Work out the finished part from the listing and answer in its coordinate system (mm). A direction names the side the tool comes from. Round coordinates to 2 decimals unless told otherwise and drop trailing zeros. Write each loop counter-clockwise with the first axis right and the second up, starting at its lowest first coordinate (ties: lowest second). Pieces come first, ordered by that corner, then holes.
1. Flat-ended cylindrical pins translate along their axes: pin 1 Ø10 at (y, z) = (67.5, 14.5) entering from +X; pin 2 Ø3 at (x, y) = (11, 97) entering from +Z; pin 3 Ø15.5 at (x, z) = (0.5, 2.5) entering from -Y; pin 4 Ø5 at (x, y) = (-11, 12.5) entering from -Z. Find the tip coordinate at first contact, or state that the pin passes through.
2. A tool of negligible diameter and unlimited length cuts with its end or side. For faces 1 (the face through (-20.93, 71.86, 17.35)), 2 (the face through (14.39, 89, -8)), 3 (the face through (5.437, 0.493, -17.264)), from which of +Z, -Z, +X, -X, +Y, -Y can it reach the whole face along a straight path? Write none if from no direction.
3. Straight lines are drawn through the part: probe 1 along X at (y, z) = (92.15, -16); probe 2 along Y at (x, z) = (-9.5, -19); probe 3 along X at (y, z) = (-3, 0). For each, find the intervals that lie inside material, in ascending order.
4. Find section D-D (y = 98). Write down the section's boundary in (x, z), and give its area (3 significant figures).
5. Find section C-C (z = 0). Count the separate pieces of the cut face and the enclosed holes in it, and give its area (3 significant figures).
6. Find section A-A (y = 79.5). Write down the section's boundary in (x, z), and give its area (3 significant figures).
7. Determine the mould class of faces 4 (the face through (2, 91, -9)), 5 (the face through (22, 83, -6)), 6 (the face through (-5, 77.5, -16)) for opening direction X: pulls with the +X half, pulls with the -X half, needs draft (parallel to the pull), parting line crosses it, or undercut.
8. Find section B-B (y = 13.5). Write down the section's boundary in (x, z).
```python
from build123d import *

# Parameters (mm, degrees)
SKETCH_1_R           = 18.6
EXTRUDE_1_DEPTH      = 15
SKETCH_2_R           = 19.1
EXTRUDE_2_DEPTH      = 43
FILLET_4_R           = 1
SKETCH_3_R           = 18.1
CUT_EXTRUDE_1_DEPTH  = 1
SKETCH_4_R           = 7.3
EXTRUDE_3_DEPTH      = 5.7
FILLET_5_R           = 1
SKETCH_5_R           = 4
CUT_EXTRUDE_2_DEPTH  = 2
SKETCH_6_R           = 2.25
EXTRUDE_4_DEPTH      = 2
SKETCH_7_R           = 7
EXTRUDE_5_DEPTH      = 4.1
SKETCH_8_R           = 6.5
CUT_EXTRUDE_3_DEPTH  = 2.6
SKETCH_9_R           = 2.5
EXTRUDE_6_DEPTH      = 3
SKETCH_10_R          = 5
EXTRUDE_7_DEPTH      = 19
SKETCH_12_W          = 44
SKETCH_12_H          = 57
EXTRUDE_8_DEPTH      = 4
SKETCH_13_R          = 3
EXTRUDE_9_DEPTH      = 20
SKETCH_14_R          = 3
EXTRUDE_10_DEPTH     = 20
SKETCH_15_R          = 3
EXTRUDE_11_DEPTH     = 20
SKETCH_16_R          = 3
EXTRUDE_12_DEPTH     = 20
SKETCH_17_W          = 44
SKETCH_17_H          = 57
EXTRUDE_13_DEPTH     = 3
SKETCH_21_R          = 6.5
SKETCH_21_R_2        = 2.5
CUT_EXTRUDE_5_DEPTH  = 4
CUT_EXTRUDE_START    = -4
SKETCH_22_R          = 7
CUT_EXTRUDE_6_DEPTH  = 4
SKETCH_23_R          = 5.5
SKETCH_23_R_2        = 4.5
EXTRUDE_14_DEPTH     = 0.1
SKETCH_24_R          = 4
EXTRUDE_15_DEPTH     = 10
SKETCH_25_R          = 5
EXTRUDE_16_DEPTH     = 3.5
SKETCH_28_R          = 10.9
EXTRUDE_22_DEPTH     = 2
SKETCH_29_R          = 4
EXTRUDE_23_DEPTH     = 4.5
EXTRUDE_START        = 0.1
SKETCH_31_R          = 5.5
SKETCH_31_R_2        = 4.5
EXTRUDE_25_DEPTH     = 0.1
EXTRUDE_26_DEPTH     = 9
CUT_EXTRUDE_7_DEPTH  = 9
CUT_EXTRUDE_8_DEPTH  = 9
SKETCH_39_R          = 2.75
EXTRUDE_27_DEPTH     = 15
CUT_EXTRUDE_9_DEPTH  = 9
SKETCH_41_W          = 1
SKETCH_41_H          = 1
CUT_EXTRUDE_10_DEPTH = 9
SKETCH_42_W          = 1
SKETCH_42_H          = 1
CUT_EXTRUDE_11_DEPTH = 9
FILLET_6_R           = 0.01
FILLET_7_R           = 0.1
SKETCH_43_R          = 7.5
SKETCH_43_R_2        = 7
CUT_EXTRUDE_12_DEPTH = 3
SKETCH_44_R          = 30
EXTRUDE_28_DEPTH     = 5


with BuildPart() as part:
    # ｽｹｯﾁ1 → ﾎﾞｽ - 押し出し1 (new body)
    with BuildSketch(Plane(origin=(0, 0, 0), x_dir=(1, 0, 0), z_dir=(0, 1, 0))):
        with Locations(Location((0, 0, 0), (0, 0, 270))):
            Circle(SKETCH_1_R)
    extrude(amount=EXTRUDE_1_DEPTH)

    # ｽｹｯﾁ2 → ﾎﾞｽ - 押し出し2 (add)
    with BuildSketch(Plane(origin=(0, 15, 0), x_dir=(1, 0, 0), z_dir=(0, 1, 0))):
        with Locations(Location((0, 0, 0), (0, 0, 270))):
            Circle(SKETCH_2_R)
    extrude(amount=EXTRUDE_2_DEPTH)

    # ﾌｨﾚｯﾄ4
    fillet_4_edges = [part.edges().sort_by_distance(p)[0] for p in [
        (0, 58, -19.1),
    ]]
    fillet(fillet_4_edges, radius=FILLET_4_R)

    # ｽｹｯﾁ3 → ｶｯﾄ - 押し出し1 (cut)
    with BuildSketch(Plane.XZ):
        with Locations(Location((0, 0, 0), (0, 0, 270))):
            Circle(SKETCH_3_R)
    extrude(amount=-CUT_EXTRUDE_1_DEPTH, mode=Mode.SUBTRACT)

    # ｽｹｯﾁ4 → ﾎﾞｽ - 押し出し3 (add)
    with BuildSketch(Plane.XZ.offset(-1)):
        with Locations(Location((0, 0, 0), (0, 0, 270))):
            Circle(SKETCH_4_R)
    extrude(amount=EXTRUDE_3_DEPTH)

    # ﾌｨﾚｯﾄ5
    fillet_5_edges = [part.edges().sort_by_distance(p)[0] for p in [
        (0, -4.7, 7.3),
    ]]
    fillet(fillet_5_edges, radius=FILLET_5_R)

    # ｽｹｯﾁ5 → ｶｯﾄ - 押し出し2 (cut)
    with BuildSketch(Plane.XZ.offset(4.7)):
        with Locations(Location((0, 0, 0), (0, 0, 270))):
            Circle(SKETCH_5_R)
    extrude(amount=-CUT_EXTRUDE_2_DEPTH, mode=Mode.SUBTRACT)

    # ｽｹｯﾁ6 → ﾎﾞｽ - 押し出し4 (add)
    with BuildSketch(Plane.XZ.offset(2.7)):
        with Locations(Location((0, 0, 0), (0, 0, 270))):
            Circle(SKETCH_6_R)
    extrude(amount=EXTRUDE_4_DEPTH)

    # ｽｹｯﾁ7 → ﾎﾞｽ - 押し出し5 (add)
    with BuildSketch(Plane(origin=(0, 58, 0), x_dir=(1, 0, 0), z_dir=(0, 1, 0))):
        with Locations(Location((0, 0, 0), (0, 0, 270))):
            Circle(SKETCH_7_R)
    extrude(amount=EXTRUDE_5_DEPTH)

    # ｽｹｯﾁ8 → ｶｯﾄ - 押し出し3 (cut)
    with BuildSketch(Plane(origin=(0, 62.1, 0), x_dir=(1, 0, 0), z_dir=(0, 1, 0))):
        with Locations(Location((0, 0, 0), (0, 0, 270))):
            Circle(SKETCH_8_R)
    extrude(amount=-CUT_EXTRUDE_3_DEPTH, mode=Mode.SUBTRACT)

    # ｽｹｯﾁ9 → ﾎﾞｽ - 押し出し6 (add)
    with BuildSketch(Plane(origin=(0, 59.5, 0), x_dir=(1, 0, 0), z_dir=(0, 1, 0))):
        with Locations(Location((0, 0, 0), (0, 0, 270))):
            Circle(SKETCH_9_R)
    extrude(amount=EXTRUDE_6_DEPTH)

    # ｽｹｯﾁ10 → ﾎﾞｽ - 押し出し7 (add)
    with BuildSketch(Plane(origin=(0, 62.5, 0), x_dir=(1, 0, 0), z_dir=(0, 1, 0))):
        with Locations(Location((0, 0, 0), (0, 0, 270))):
            Circle(SKETCH_10_R)
    extrude(amount=EXTRUDE_7_DEPTH)

    # ｽｹｯﾁ12 → ﾎﾞｽ - 押し出し8 (add)
    with BuildSketch(Plane(origin=(0, 58, 0), x_dir=(1, 0, 0), z_dir=(0, 1, 0))):
        with Locations((0, 6.5)):
            Rectangle(SKETCH_12_W, SKETCH_12_H)
    extrude(amount=EXTRUDE_8_DEPTH)

    # ｽｹｯﾁ13 → ﾎﾞｽ - 押し出し9 (add)
    with BuildSketch(Plane(origin=(0, 62, 0), x_dir=(1, 0, 0), z_dir=(0, 1, 0))):
        with Locations(Location((-18, 31, 0), (0, 0, 270))):
            Circle(SKETCH_13_R)
    extrude(amount=EXTRUDE_9_DEPTH)

    # ｽｹｯﾁ14 → ﾎﾞｽ - 押し出し10 (add)
    with BuildSketch(Plane(origin=(0, 62, 0), x_dir=(1, 0, 0), z_dir=(0, 1, 0))):
        with Locations(Location((-18, -18, 0), (0, 0, 270))):
            Circle(SKETCH_14_R)
    extrude(amount=EXTRUDE_10_DEPTH)

    # ｽｹｯﾁ15 → ﾎﾞｽ - 押し出し11 (add)
    with BuildSketch(Plane(origin=(0, 62, 0), x_dir=(1, 0, 0), z_dir=(0, 1, 0))):
        with Locations(Location((18, 31, 0), (0, 0, 270))):
            Circle(SKETCH_15_R)
    extrude(amount=EXTRUDE_11_DEPTH)

    # ｽｹｯﾁ16 → ﾎﾞｽ - 押し出し12 (add)
    with BuildSketch(Plane(origin=(0, 62, 0), x_dir=(1, 0, 0), z_dir=(0, 1, 0))):
        with Locations(Location((18, -18, 0), (0, 0, 270))):
            Circle(SKETCH_16_R)
    extrude(amount=EXTRUDE_12_DEPTH)

    # ｽｹｯﾁ17 → ﾎﾞｽ - 押し出し13 (add)
    with BuildSketch(Plane(origin=(0, 82, 0), x_dir=(1, 0, 0), z_dir=(0, 1, 0))):
        with Locations((0, 6.5)):
            Rectangle(SKETCH_17_W, SKETCH_17_H)
    extrude(amount=EXTRUDE_13_DEPTH)

    # ｽｹｯﾁ21 → ｶｯﾄ - 押し出し5 (cut)
    with BuildSketch(Plane(origin=(0, 62, 0), x_dir=(1, 0, 0), z_dir=(0, 1, 0))):
        with Locations(Location((0, 0, 0), (0, 0, 270))):
            Circle(SKETCH_21_R)
        with Locations(Location((0, 0, 0), (0, 0, 270))):
            Circle(SKETCH_21_R_2, mode=Mode.SUBTRACT)
    extrude(amount=-CUT_EXTRUDE_5_DEPTH, mode=Mode.SUBTRACT)

    # ｽｹｯﾁ22 → ｶｯﾄ - 押し出し6 (cut)
    with BuildSketch(Plane(origin=(0, 85, 0), x_dir=(1, 0, 0), z_dir=(0, 1, 0)).offset(CUT_EXTRUDE_START)):
        with Locations(Location((0, 0, 0), (0, 0, 270))):
            Circle(SKETCH_22_R)
    extrude(amount=CUT_EXTRUDE_6_DEPTH, mode=Mode.SUBTRACT)

    # ｽｹｯﾁ23 → ﾎﾞｽ - 押し出し14 (add)
    with BuildSketch(Plane(origin=(0, 62, 0), x_dir=(1, 0, 0), z_dir=(0, 1, 0))):
        with Locations(Location((0, 16, 0), (0, 0, 270))):
            Circle(SKETCH_23_R)
        with Locations(Location((0, 16, 0), (0, 0, 270))):
            Circle(SKETCH_23_R_2, mode=Mode.SUBTRACT)
    extrude(amount=EXTRUDE_14_DEPTH)

    # ｽｹｯﾁ24 → ﾎﾞｽ - 押し出し15 (add)
    with BuildSketch(Plane(origin=(0, 62, 0), x_dir=(1, 0, 0), z_dir=(0, 1, 0))):
        with Locations(Location((0, 16, 0), (0, 0, 270))):
            Circle(SKETCH_24_R)
    extrude(amount=EXTRUDE_15_DEPTH)

    # ｽｹｯﾁ25 → ﾎﾞｽ - 押し出し16 (add)
    with BuildSketch(Plane(origin=(0, 72, 0), x_dir=(1, 0, 0), z_dir=(0, 1, 0))):
        with Locations(Location((0, 16, 0), (0, 0, 270))):
            Circle(SKETCH_25_R)
    extrude(amount=EXTRUDE_16_DEPTH)

    # ｽｹｯﾁ28 → ﾎﾞｽ - 押し出し22 (add)
    with BuildSketch(Plane(origin=(0, 75.5, 0), x_dir=(1, 0, 0), z_dir=(0, 1, 0))):
        with Locations(Location((0, 16, 0), (0, 0, 270))):
            Circle(SKETCH_28_R)
    extrude(amount=EXTRUDE_22_DEPTH)

    # ｽｹｯﾁ29 → ﾎﾞｽ - 押し出し23 (add)
    with BuildSketch(Plane(origin=(0, 77.5, 0), x_dir=(1, 0, 0), z_dir=(0, 1, 0))):
        with Locations(Location((0, 16, 0), (0, 0, 270))):
            Circle(SKETCH_29_R)
    extrude(amount=EXTRUDE_23_DEPTH)

    # ｽｹｯﾁ31 → ﾎﾞｽ - 押し出し25 (add)
    with BuildSketch(Plane.XZ.offset(-82).offset(EXTRUDE_START)):
        with Locations(Location((0, -16, 0), (0, 0, 90))):
            Circle(SKETCH_31_R)
        with Locations(Location((0, -16, 0), (0, 0, 90))):
            Circle(SKETCH_31_R_2, mode=Mode.SUBTRACT)
    extrude(amount=-EXTRUDE_25_DEPTH)

    # ｽｹｯﾁ32 → ﾎﾞｽ - 押し出し26 (add)
    with BuildSketch(Plane(origin=(0, 85, 0), x_dir=(1, 0, 0), z_dir=(0, 1, 0))):
        with BuildLine():
            Line((-14.38, 23.72089526), (-14.38, 14.139608929))
            Line((-14.38, 14.139608929), (-14.38, -11.913385086))
            Line((-14.38, -11.913385086), (14.39, -11.913385086))
            Line((14.39, -11.913385086), (14.39, 14.139608929))
            Line((14.39, 14.139608929), (14.39, 24.129341302))
            ThreePointArc((14.39, 24.129341302), (-0.101833491, 31.450223746), (-14.38, 23.72089526))
        make_face()
    extrude(amount=EXTRUDE_26_DEPTH)

    # ｽｹｯﾁ35 → ｶｯﾄ - 押し出し7 (cut)
    with BuildSketch(Plane(origin=(0, 94, 0), x_dir=(1, 0, 0), z_dir=(0, 1, 0))):
        Polygon((14.39, -11.913385086), (14.39, -7.913385086), (9.39, -11.913385086), align=None)
    extrude(amount=-CUT_EXTRUDE_7_DEPTH, mode=Mode.SUBTRACT)

    # ｽｹｯﾁ37 → ｶｯﾄ - 押し出し8 (cut)
    with BuildSketch(Plane(origin=(0, 94, 0), x_dir=(1, 0, 0), z_dir=(0, 1, 0))):
        Polygon((-14.38, -11.913385086), (-9.38, -11.913385086), (-14.38, -7.913385086), align=None)
    extrude(amount=-CUT_EXTRUDE_8_DEPTH, mode=Mode.SUBTRACT)

    # ｽｹｯﾁ39 → ﾎﾞｽ - 押し出し27 (add)
    with BuildSketch(Plane(origin=(0, 94, 0), x_dir=(1, 0, 0), z_dir=(0, 1, 0))):
        with Locations(Location((0, 16, 0), (0, 0, 90))):
            Circle(SKETCH_39_R)
    extrude(amount=EXTRUDE_27_DEPTH)

    # ｽｹｯﾁ40 → ｶｯﾄ - 押し出し9 (cut)
    with BuildSketch(Plane.XY.offset(11.913385086)):
        Polygon((-8, 90), (-3.5, 90), (-3.5, 91.5), (3.5, 91.5), (3.5, 90), (8, 90), (8, 87), (-8, 87), align=None)
    extrude(amount=-CUT_EXTRUDE_9_DEPTH, mode=Mode.SUBTRACT)

    # ｽｹｯﾁ41 → ｶｯﾄ - 押し出し10 (cut)
    with BuildSketch(Plane.XY.offset(11.913385086)):
        with Locations((3, 86.5)):
            Rectangle(SKETCH_41_W, SKETCH_41_H)
    extrude(amount=-CUT_EXTRUDE_10_DEPTH, mode=Mode.SUBTRACT)

    # ｽｹｯﾁ42 → ｶｯﾄ - 押し出し11 (cut)
    with BuildSketch(Plane.XY.offset(11.913385086)):
        with Locations((-4, 86.5)):
            Rectangle(SKETCH_42_W, SKETCH_42_H)
    extrude(amount=-CUT_EXTRUDE_11_DEPTH, mode=Mode.SUBTRACT)

    # ﾌｨﾚｯﾄ6
    fillet_6_edges = [part.edges().sort_by_distance(p)[0] for p in [
        (0, 109, -13.25),
    ]]
    fillet(fillet_6_edges, radius=FILLET_6_R)

    # ﾌｨﾚｯﾄ7
    fillet_7_edges = [part.edges().sort_by_distance(p)[0] for p in [
        (14.39, 89.5, -24.129341302),
        (-14.38, 89.5, -23.72089526),
        (14.39, 89.5, 7.913385086),
        (9.39, 89.5, 11.913385086),
        (-14.38, 89.5, 7.913385086),
        (-9.38, 89.5, 11.913385086),
    ]]
    fillet(fillet_7_edges, radius=FILLET_7_R)

    # ｽｹｯﾁ43 → ｶｯﾄ - 押し出し12 (cut)
    with BuildSketch(Plane(origin=(0, 94, 0), x_dir=(1, 0, 0), z_dir=(0, 1, 0))):
        with Locations(Location((0, 16, 0), (0, 0, 270))):
            Circle(SKETCH_43_R)
        with Locations(Location((0, 16, 0), (0, 0, 270))):
            Circle(SKETCH_43_R_2, mode=Mode.SUBTRACT)
    extrude(amount=-CUT_EXTRUDE_12_DEPTH, mode=Mode.SUBTRACT)

    # ｽｹｯﾁ44 → ﾎﾞｽ - 押し出し28 (add)
    with BuildSketch(Plane(origin=(0, 109, 0), x_dir=(1, 0, 0), z_dir=(0, 1, 0))):
        with Locations(Location((0, 16, 0), (0, 0, 270))):
            Circle(SKETCH_44_R)
    extrude(amount=-EXTRUDE_28_DEPTH)


solid = part.part
```
Worked answers:
1. pin 1: stops at x = 21
1. pin 2: passes through
1. pin 3: stops at y = -4.7
1. pin 4: stops at z = -16.54
2. face 1: none
2. face 2: +Z, -Z, +X
2. face 3: -Y
3. probe 1: x = -14.38 to -7.5, -7 to 7, 7.5 to 14.39
3. probe 2: y = 58 to 62, 75.5 to 77.5, 82 to 94, 104 to 109
3. probe 3: x = -7.3 to -4, -2.25 to 2.25, 4 to 7.3
4. outline: circle Ø5.5 at (0, -16)
4. area: 23.8 mm2
5. separate pieces: 3
5. enclosed holes: 0
5. area: 3,170 mm2
6. outline: circle Ø6 at (-18, -31); circle Ø6 at (-18, 18); circle Ø10 at (0, 0); circle Ø8 at (0, -16); circle Ø6 at (18, -31); circle Ø6 at (18, 18)
6. area: 242 mm2
7. face 4: undercut
7. face 5: pulls with the +X half
7. face 6: needs draft
8. outline: circle Ø37.2 at (0, 0)
